Here's how the part is built. I have some questions about the finished solid (model axes, mm). Face numbers are marked on the shaded views. A direction names the side the tool comes from. Round coordinates to 2 decimals unless told otherwise and drop trailing zeros. Write each loop counter-clockwise with the first axis right and the second up, starting at its lowest first coordinate (ties: lowest second). Pieces come first, ordered by that corner, then holes. Notation, with made-up numbers: M -9,65 L 25,65 A33 cw 25,100 Z; hole C 86.25,66 d7. An arc over 180 degrees is marked long. Use one line per item in the form item = value. Start each with the question number.
Q1. I want a section at C-C on y = 7.5. List the corners of the cut face in (x, z) for me.
Q2. I'm going to push flat-ended pins straight in: pin 1 Ø3.5 at (x, y) = (22.5, 6) entering from +Z; pin 2 Ø1.5 at (y, z) = (6, 12.5) entering from -X. Where does each tip first touch, or does it pass through?
Q3. We'd pull the mould along X, two halves only. Please class the marked faces 6, 7, 8 and 9: +X half, -X half, draft (parallel to the pull), parting line (faces both ways), or undercut.
Q4. I want a section at B-B on z = 6.5. State how many separate pieces and enclosed holes the cut face has, and give its area (3 significant figures).
Q5. I want a section at D-D on z = 12. List the corners of the cut face in (x, y) for me.
Q6. I want a section at A-A on x = 24. List the corners of the cut face in (y, z) for me.
Q7. I need wall thicknesses on line 1 along X through (y, z) = (5.5, 4.25); line 2 along Y through (x, z) = (18, 8.5); line 3 along X through (y, z) = (3.5, 8). Which ranges of each line are inside material? Lowest first, please. Write a range as from..to.
Q8. For the marked faces 1, 2, 3, 4 and 5, which set-ups out of +Z, -Z, +X, -X, +Y, -Y let a thin tool reach every point of the face, with its end or its side?
```python
from build123d import *

# Parameters (mm, degrees)
F0_W     = 30
F0_H     = 11
F1_DEPTH = 9
F2_W     = 11
F2_H     = 11
F3_DEPTH = 5
F4_R     = 1.5
F5_R     = 5.49999
F6_W     = 7
F6_H     = 7
F7_DEPTH = 25
F9_DEPTH = 25


# Not quite as in the source:
# - a fillet or chamfer is up to 0.001 mm smaller than in the source, because OpenCascade refuses the exact size


with BuildPart() as f1:
    # F0 (on Top) → F1 (new body)
    with BuildSketch(Plane.XY):
        with Locations((15, 5.5)):
            Rectangle(F0_W, F0_H)
    extrude(amount=F1_DEPTH)

    # F2 (on face) → F3 (join)
    with BuildSketch(Plane.XY.offset(9)):
        with Locations((15, 5.5)):
            Rectangle(F2_W, F2_H)
    extrude(amount=F3_DEPTH)

    # F4
    f4_edges = [f1.edges().sort_by_distance(p)[0] for p in [
        (20.5, 11, 11.5),
        (9.5, 11, 11.5),
        (9.5, 0, 11.5),
        (20.5, 0, 11.5),
    ]]
    fillet(f4_edges, radius=F4_R)

    # F5 (radius 5.5 in the source; OpenCascade refuses exactly that, so slightly less here)
    f5_edges = [f1.edges().sort_by_distance(p)[0] for p in [
        (30, 11, 4.5),
        (30, 0, 4.5),
        (0, 11, 4.5),
        (0, 0, 4.5),
    ]]
    fillet(f5_edges, radius=F5_R)

    # F6 (on face) → F7 (cut)
    with BuildSketch(Plane.XY.offset(14)):
        with Locations((15, 5.5)):
            Rectangle(F6_W, F6_H)
    extrude(amount=-F7_DEPTH, mode=Mode.SUBTRACT)

    # F8 (on face) → F9 (cut)
    with BuildSketch(Plane.XY.offset(9)):
        with BuildLine():
            Line((24.5, 9), (22.5, 9))
            Line((22.5, 9), (22.5, 2))
            Line((22.5, 2), (24.5, 2))
            ThreePointArc((24.5, 2), (28, 5.5), (24.5, 9))
        make_face()
        with BuildLine():
            Line((7.5, 2), (7.5, 9))
            Line((7.5, 9), (5.5, 9))
            ThreePointArc((5.5, 9), (2, 5.5), (5.5, 2))
            Line((5.5, 2), (7.5, 2))
        make_face()
    extrude(amount=-F9_DEPTH, mode=Mode.SUBTRACT)


solid = f1.part
```
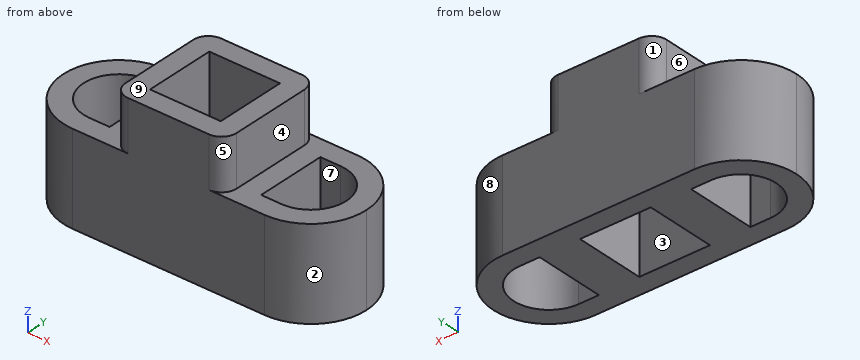
Reported:
q1.outline = M 0.38,0 L 2.63,0 L 2.63,9 L 0.38,9 Z; M 7.5,0 L 11.5,0 L 11.5,14 L 9.5,14 L 9.5,9 L 7.5,9 Z; M 18.5,0 L 22.5,0 L 22.5,9 L 20.5,9 L 20.5,14 L 18.5,14 Z; M 27.37,0 L 29.62,0 L 29.62,9 L 27.37,9 Z
q2.pin_1 = 9
q2.pin_2 = 9.5
q3.face_6 = -X half
q3.face_7 = undercut
q3.face_8 = +X half
q3.face_9 = draft
q4.separate_pieces = 1
q4.enclosed_holes = 3
q4.area = 189 mm^2
q5.outline = M 9.5,1.5 A1.5 ccw 11,0 L 19,0 A1.5 ccw 20.5,1.5 L 20.5,9.5 A1.5 ccw 19,11 L 11,11 A1.5 ccw 9.5,9.5 Z; hole M 11.5,2 L 18.5,2 L 18.5,9 L 11.5,9 Z
q6.outline = M 0,0 L 2,0 L 2,9 L 0,9 Z; M 9,0 L 11,0 L 11,9 L 9,9 Z
q7.line_1 = 0..2, 7.5..11.5, 18.5..22.5, 28..30
q7.line_2 = 0..2, 9..11
q7.line_3 = 0.38..2.63, 7.5..11.5, 18.5..22.5, 27.37..29.62
q8.face_1 = +Z, -X, +Y
q8.face_2 = +Z, -Z, +X, -Y
q8.face_3 = +Z, -Z
q8.face_4 = +Z, +X, +Y, -Y
q8.face_5 = +Z, +X, -Y
